```python
from build123d import *

# Parameters (mm, degrees)
SKETCH1_R           = 1.5
BOSS_EXTRUDE1_DEPTH = 3


with BuildPart() as part:
    # Sketch1 → Boss-Extrude1 (new body)
    with BuildSketch(Plane.XY):
        with BuildLine():
            Line((0, 5), (19.85, 5))
            Line((19.85, 5), (44.643069029, 15.193663072))
            ThreePointArc((44.643069029, 15.193663072), (45.042006379, 15.268610471), (45.43786686, 15.178818479))
            Line((45.43786686, 15.178818479), (51.245085043, 12.533540635))
            ThreePointArc((51.245085043, 12.533540635), (51.550738574, 12.317286013), (51.755428853, 12.003770413))
            Line((51.755428853, 12.003770413), (52.954960556, 9.086264498))
            Line((52.954960556, 9.086264498), (53.647413738, 7.201821951))
            Line((53.647413738, 7.201821951), (53.200417763, 6.109762155))
            Line((53.200417763, 6.109762155), (51.987413738, 6.606262365))
            Line((51.987413738, 6.606262365), (51.540417763, 5.514202569))
            Line((51.540417763, 5.514202569), (50.327413738, 6.010702778))
            Line((50.327413738, 6.010702778), (49.901790908, 4.970859901))
            Line((49.901790908, 4.970859901), (48.688786884, 5.467360111))
            Line((48.688786884, 5.467360111), (48.241790908, 4.375300315))
            Line((48.241790908, 4.375300315), (47.028786884, 4.871800524))
            Line((47.028786884, 4.871800524), (46.581790908, 3.779740729))
            Line((46.581790908, 3.779740729), (40.742047423, 6.170032768))
            Line((40.742047423, 6.170032768), (28.174379319, 1.158584034))
            Line((28.174379319, 1.158584034), (24, -5))
            Line((24, -5), (22, -5))
            Line((22, -5), (0, -5))
            ThreePointArc((0, -5), (-5, 0), (0, 5))
        make_face()
        Circle(SKETCH1_R, mode=Mode.SUBTRACT)
        with Locations((22, 0)):
            Circle(SKETCH1_R, mode=Mode.SUBTRACT)
    extrude(amount=BOSS_EXTRUDE1_DEPTH)


solid = part.part
```
Here's how the part is built. I have some questions about the finished solid (model axes, mm). A direction names the side the tool comes from. Round coordinates to 2 decimals unless told otherwise and drop trailing zeros. Write each loop counter-clockwise with the first axis right and the second up, starting at its lowest first coordinate (ties: lowest second). Pieces come first, ordered by that corner, then holes.
Q1. Will this pin go through, and if not, where does the flat tip stop? P1, Ø1.5, axis at x = 12, z = 1, coming from the +Y side.
Q2. If we section it at A-A on x = 1: Write out the boundary of the cut face in (y, z).
Q3. If we section it at D-D on x = 22: Write out the boundary of the cut face in (y, z), plus the area to 3 significant figures.
Q4. If we section it at C-C on z = 2.05: Write out the boundary of the cut face in (x, y).
Q5. If we mould it in two halves opening along Y, with no side actions, what happens to faces 1 (the flat face through (10, 5, 1)), 2 (the cylindrical face through (-5, 0, 1)), 3 (the flat face through (50.94, 5.76, 1.48)), 4 (the cylindrical face through (-1.5, 0.07, 1.48))? For each: +Y half, -Y half, draft (parallel to the pull), parting line (faces both ways), or undercut.
Q6. Which directions (+Z, -Z, +X, -X, +Y, -Y) give clear straight access to the entire face, cutting with the end or side of a thin tool? Please do faces 5 (the flat face through (46.808, 4.333, 1.479)), 6 (the cylindrical face through (20.5, 0.07, 1.48)).
Q7. Please list where these lines run through material, in increasing order: probe 1 along Y at (x, z) = (0, 2.4); probe 2 along X at (y, z) = (0.5, 2.95); probe 3 along Y at (x, z) = (22, 1.55).
Q8. If we section it at B-B on y = 0: Write out the boundary of the cut face in (x, z), plus the area to 3 significant figures.
Answer below:
1. P1: stops at y = 5
2. outline: (-5, 0) - (-1.12, 0) - (-1.12, 3) - (-5, 3) - close; (1.12, 0) - (5, 0) - (5, 3) - (1.12, 3) - close
3. outline: (-5, 0) - (-1.5, 0) - (-1.5, 3) - (-5, 3) - close; (1.5, 0) - (5.88, 0) - (5.88, 3) - (1.5, 3) - close
3. area: 23.7 mm2
4. outline: (0, -5) - (24, -5) - (28.17, 1.16) - (40.74, 6.17) - (46.58, 3.78) - (47.03, 4.87) - (48.24, 4.38) - (48.69, 5.47) - (49.9, 4.97) - (50.33, 6.01) - (51.54, 5.51) - (51.99, 6.61) - (53.2, 6.11) - (53.65, 7.2) - (52.95, 9.09) - (51.76, 12) arc R1 ccw to (51.25, 12.53) - (45.44, 15.18) arc R1 ccw to (44.64, 15.19) - (19.85, 5) - (0, 5) arc R5 ccw to start; hole circle Ø3 at (0, 0); hole circle Ø3 at (22, 0)
5. face 1: +Y half
5. face 2: parting line
5. face 3: -Y half
5. face 4: undercut
6. face 5: +Z, -Z, -Y
6. face 6: +Z, -Z
7. probe 1: y = -5 to -1.5, 1.5 to 5
7. probe 2: x = -4.97 to -1.41, 1.41 to 20.59, 23.41 to 27.73
7. probe 3: y = -5 to -1.5, 1.5 to 5.88
8. outline: (-5, 0) - (-1.5, 0) - (-1.5, 3) - (-5, 3) - close; (1.5, 0) - (20.5, 0) - (20.5, 3) - (1.5, 3) - close; (23.5, 0) - (27.39, 0) - (27.39, 3) - (23.5, 3) - close
8. area: 79.2 mm2
